Autodesk Inventor part; units mm, degrees
ref_plane "YZ Plane" through (0, 0, 0) normal (1, 0, 0) x (0, 1, 0)
ref_plane "XZ Plane" through (0, 0, 0) normal (0, 1, 0) x (-1, 0, 0)
ref_plane "XY Plane" through (0, 0, 0) normal (0, 0, 1) x (1, 0, 0)
sketch "Sketch1" plane through (0, 0, 0) normal (0, 0, 1) x (1, 0, 0)
  line L0 (0, 0) -> (26.6192, 0)
  line L1 (26.6192, 0) -> (26.6192, 47.0916)
  line L2 (26.6192, 47.0916) -> (0, 47.0916)
  line L3 (0, 47.0916) -> (0, 0)
  dimension "d0" = 26.6192
  dimension "d1" = 47.0916
extrude "Extrusion1" add sketch "Sketch1" along normal blind 3.175
sketch "Sketch6" plane through (26.6192, 0, 0) normal (1, 0, 0) x (0, 0, -1)
  line L0 (0, 0) -> (-10.7442, 0)
  line L1 (-10.7442, 0) -> (-10.7442, 47.0916)
  line L2 (-10.7442, 47.0916) -> (0, 47.0916)
  line L3 (0, 47.0916) -> (0, 0)
  dimension "d15" = 10.7442
extrude "Extrusion6" add sketch "Sketch6" along normal blind 42.0116
sketch "Sketch7" plane through (68.6308, 0, 0) normal (1, 0, 0) x (0, 0, -1)
  line L0 (0, 47.0916) -> (0, 0)
  line L1 (-3.175, 47.0916) -> (-3.175, 0)
  line L2 (0, 0) -> (-3.175, 0)
  line L3 (-3.175, 0) -> (-3.175, 47.0916)
  line L4 (-3.175, 47.0916) -> (0, 47.0916)
  line L5 (0, 47.0916) -> (0, 0)
extrude "Extrusion7" add sketch "Sketch7" along normal blind 26.6192
properties part number "bagcimspacer" material "Aluminum 6061"
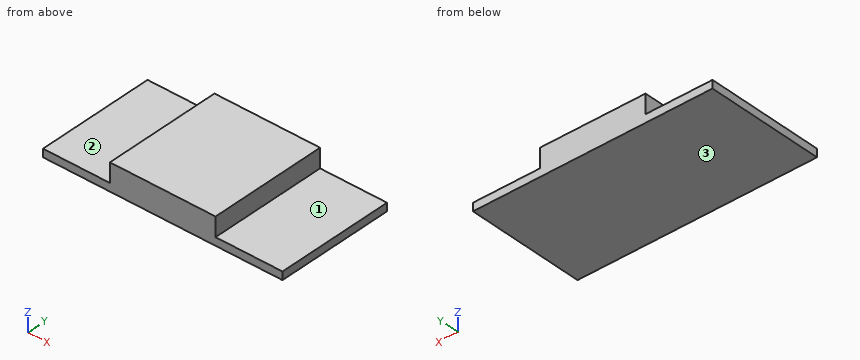
Can you work these out from the model? Positions are in its coordinate system, mm. Face numbers are marked on the shaded views. A direction names the side the tool comes from. Coordinates: 2 decimals unless noted, no trailing zeros. Loops run counter-clockwise (first coordinate to the right, second up) from the corner with the lowest first, then second, coordinate; pieces in that order, holes last.
Item 1: I'm going to push flat-ended pins straight in: pin 1 (2.5 mm diameter, centred on y = 24.5, z = 7, fed in from -X); pin 2 (5 mm diameter, centred on x = 21.5, z = 8, fed in from -Y); pin 3 (21.5 mm diameter, centred on x = 14.5, y = 26.5, fed in from +Z) (3 decimals); pin 4 (4 mm diameter, centred on y = 26.5, z = 7, fed in from +X). Where does each tip first touch, or does it pass through?
Answers below:
pin 1: stops at x = 26.62
pin 2: passes through
pin 3: stops at z = 3.175
pin 4: stops at x = 68.63
Item 2: Suppose I cut it at B-B (z = 4.25). Please give me the cut outline in (x, y), then the cut area to 3 significant figures.
Answers below:
outline: (26.62, 0) - (68.63, 0) - (68.63, 47.09) - (26.62, 47.09) - close
area: 1,980 mm2
Item 3: Suppose I cut it at A-A (y = 6). Please give me the cut outline in (x, z) (3 decimals), then the cut area to 3 significant figures.
Answers below:
outline: (0, 0) - (95.25, 0) - (95.25, 3.175) - (68.631, 3.175) - (68.631, 10.744) - (26.619, 10.744) - (26.619, 3.175) - (0, 3.175) - close
area: 620 mm2
Item 4: Which directions (+Z, -Z, +X, -X, +Y, -Y) give clear straight access to the entire face, cutting with the end or side of a thin tool? Please do the marked faces 1, 2 and 3.
Answers below:
face 1: +Z, +X, +Y, -Y
face 2: +Z, -X, +Y, -Y
face 3: -Z, +X, -X, +Y, -Y
Item 5: Suppose I cut it at C-C (x = 78). Please give me the cut outline in (y, z) (3 decimals), then the cut area to 3 significant figures.
Answers below:
outline: (0, 0) - (47.092, 0) - (47.092, 3.175) - (0, 3.175) - close
area: 150 mm2
Item 6: Please list where these lines run through material, in increasing order: L1, parallel to X at y = 12, z = 8.25; L2, parallel to Z at x = 22, y = 41 (3 decimals).
Answers below:
L1: x = 26.62 to 68.63
L2: z = 0 to 3.175
